```python
from build123d import *

# Parameters (mm, degrees)
SKETCH1_R           = 2.65
SKETCH1_R_2         = 4
BOSS_EXTRUDE1_DEPTH = 4.5
SKETCH2_R           = 13.25
SKETCH2_R_2         = 4
BOSS_EXTRUDE2_DEPTH = 4
SKETCH3_R           = 6
SKETCH3_R_2         = 4
BOSS_EXTRUDE3_DEPTH = 2.5
SKETCH4_R           = 11.75
SKETCH4_R_2         = 6
CUT_EXTRUDE1_DEPTH  = 1


with BuildPart() as part:
    # Sketch1 → Boss-Extrude1 (new body)
    with BuildSketch(Plane(origin=(0, 0, 0), x_dir=(1, 0, 0), z_dir=(0, 1, 0))):
        with BuildLine():
            Line((6.205696203, 11.706913967), (21.623417722, 3.534162707))
            ThreePointArc((21.623417722, 3.534162707), (23.75, 0), (21.623417722, -3.534162707))
            Line((21.623417722, -3.534162707), (6.205696203, -11.706913967))
            ThreePointArc((6.205696203, -11.706913967), (0, -13.25), (-6.205696203, -11.706913967))
            Line((-6.205696203, -11.706913967), (-21.623417722, -3.534162707))
            ThreePointArc((-21.623417722, -3.534162707), (-23.75, 0), (-21.623417722, 3.534162707))
            Line((-21.623417722, 3.534162707), (-6.205696203, 11.706913967))
            ThreePointArc((-6.205696203, 11.706913967), (0, 13.25), (6.205696203, 11.706913967))
        make_face()
        with Locations((-18.3, 0)):
            Circle(SKETCH1_R, mode=Mode.SUBTRACT)
        with Locations((18.3, 0)):
            Circle(SKETCH1_R, mode=Mode.SUBTRACT)
        Circle(SKETCH1_R_2, mode=Mode.SUBTRACT)
    extrude(amount=BOSS_EXTRUDE1_DEPTH)

    # Sketch2 → Boss-Extrude2 (add)
    with BuildSketch(Plane(origin=(0, 4.5, 0), x_dir=(1, 0, 0), z_dir=(0, 1, 0))):
        Circle(SKETCH2_R)
        Circle(SKETCH2_R_2, mode=Mode.SUBTRACT)
    extrude(amount=BOSS_EXTRUDE2_DEPTH)

    # Sketch3 → Boss-Extrude3 (add)
    with BuildSketch(Plane(origin=(0, 8.5, 0), x_dir=(1, 0, 0), z_dir=(0, 1, 0))):
        Circle(SKETCH3_R)
        Circle(SKETCH3_R_2, mode=Mode.SUBTRACT)
    extrude(amount=BOSS_EXTRUDE3_DEPTH)

    # Sketch4 → Cut-Extrude1 (cut)
    with BuildSketch(Plane(origin=(0, 8.5, 0), x_dir=(1, 0, 0), z_dir=(0, 1, 0))):
        Circle(SKETCH4_R)
        Circle(SKETCH4_R_2, mode=Mode.SUBTRACT)
    extrude(amount=-CUT_EXTRUDE1_DEPTH, mode=Mode.SUBTRACT)


solid = part.part
```
Can you work these out from the model? Positions are in its coordinate system, mm. A direction names the side the tool comes from. Coordinates: 2 decimals unless noted, no trailing zeros. Write each loop counter-clockwise with the first axis right and the second up, starting at its lowest first coordinate (ties: lowest second). Pieces come first, ordered by that corner, then holes. Notation, with made-up numbers: M 39,85.25 L 92,85.25 A33 cw 92,116.25 Z; hole C 30.5,-1.75 d6. An arc over 180 degrees is marked long. Write item = value, one per line. Start each with the question number.
Q1. If we section it at C-C, the plane x = 0: Write out the boundary of the cut face in (y, z).
Q2. If we section it at B-B, the plane y = 3.75: Write out the boundary of the cut face in (x, z), then the cut area to 3 significant figures.
Q3. On a 3-axis mill with a long thin cutter (end or side, diameter ignored), from which of +Z, -Z, +X, -X, +Y, -Y can I reach the whole of each face in a straight line? I mean faces 1 (the face through (-13.807, 2.218, 7.678)), 2 (the face through (-1, 8.5, 12)). Say none if no direction works.
Q4. Thinking about a two-plate mould opening in Z: for faces 3 (the face through (-14.022, 2.218, -7.563)), 4 (the face through (-1.42, 11, 3.92)), 5 (the face through (11.207, 8.007, -3.529)), 6 (the face through (5, 7.5, 5)), which applies, released by +Z, released by -Z, zero draft, split by the parting line, or undercut?
Q5. I'm going to push flat-ended pins straight in: pin 1 (8 mm diameter, centred on x = 16.5, z = 4.5, fed in from +Y); pin 2 (6 mm diameter, centred on y = 2.5, z = 7, fed in from +X); pin 3 (6 mm diameter, centred on x = -18.3, z = 0, fed in from +Y); pin 4 (4 mm diameter, centred on x = -15, z = -10, fed in from -Y). Where does each tip first touch, or does it pass through?
Q6. If we section it at D-D, the plane y = 9: Write out the boundary of the cut face in (x, z), then the cut area to 3 significant figures.
Q7. If I drill on L1, parallel to X at y = 1.9, z = 0; L2, parallel to Z at x = 0, y = 8.1; L3, parallel to Z at x = 0, y = 4.25, over which ranges is the centre line in solid material (lowest first)? Write a range as [from, to].
Q8. If we section it at A-A, the plane z = 0: Write out the boundary of the cut face in (x, y), then the cut area to 3 significant figures.
Check sheet entries:
q1.outline = M 0,-13.25 L 8.5,-13.25 L 8.5,-11.75 L 7.5,-11.75 L 7.5,-6 L 11,-6 L 11,-4 L 0,-4 Z; M 0,4 L 11,4 L 11,6 L 7.5,6 L 7.5,11.75 L 8.5,11.75 L 8.5,13.25 L 0,13.25 Z
q2.outline = M -21.62,-3.53 L -6.21,-11.71 A13.25 ccw 6.21,-11.71 L 21.62,-3.53 A4 ccw 21.62,3.53 L 6.21,11.71 A13.25 ccw -6.21,11.71 L -21.62,3.53 A4 ccw Z; hole C -18.3,0 d5.3; hole C 0,0 d8; hole C 18.3,0 d5.3
q2.area = 713 mm²
q3.face_1 = +Z, -X, +Y, -Y
q3.face_2 = +Y
q4.face_3 = released by -Z
q4.face_4 = zero draft
q4.face_5 = undercut
q4.face_6 = undercut
q5.pin_1 = 8.5
q5.pin_2 = 20.74
q5.pin_3 = 4.5
q5.pin_4 = through
q6.outline = C 0,0 d12; hole C 0,0 d8
q6.area = 62.8 mm²
q7.L1 = [-23.75, -20.95], [-15.65, -4], [4, 15.65], [20.95, 23.75]
q7.L2 = [-13.25, -11.75], [-6, -4], [4, 6], [11.75, 13.25]
q7.L3 = [-13.25, -4], [4, 13.25]
q8.outline = M -23.75,0 L -20.95,0 L -20.95,4.5 L -23.75,4.5 Z; M -15.65,0 L -4,0 L -4,11 L -6,11 L -6,7.5 L -11.75,7.5 L -11.75,8.5 L -13.25,8.5 L -13.25,4.5 L -15.65,4.5 Z; M 4,0 L 15.65,0 L 15.65,4.5 L 13.25,4.5 L 13.25,8.5 L 11.75,8.5 L 11.75,7.5 L 6,7.5 L 6,11 L 4,11 Z; M 20.95,0 L 23.75,0 L 23.75,4.5 L 20.95,4.5 Z
q8.area = 203 mm²
